Part model, mm, in its own coordinate system. A direction names the side the tool comes from. Round coordinates to 2 decimals unless told otherwise and drop trailing zeros. Loops run counter-clockwise (first coordinate to the right, second up) from the corner with the lowest first, then second, coordinate; pieces in that order, holes last.
(1) Probe probe 1 along Z at (x, y) = (148, 49.5) (3 decimals); probe 2 along Y at (x, z) = (171, -106); probe 3 along X at (y, z) = (-129, -416.5). List the from-to ranges inside material, lowest first.
(2) Cut at D-D on x = -84.5. List the corners of the cut face in (y, z) (3 decimals).
(3) Cut at C-C on z = -372.5. List the corners of the cut face in (x, y) (3 decimals), then the cut area to 3 significant figures.
(4) Cut at A-A on y = 0. List the corners of the cut face in (x, z) (3 decimals), then the cut area to 3 significant figures.
(5) Cut at B-B on z = -14.5. List the corners of the cut face in (x, y), then the cut area to 3 significant figures.
(6) Mould opens along X. For faces 1 (the face through (-228.6, -3, -308)), 2 (the face through (-118, 208.915, -504)), 3 (the face through (-86.949, -195.196, -145.643)), 4 (the face through (-84.531, -195.196, -471.703)) say: +X half, -X half, draft (parallel to the pull), parting line (faces both ways), or undercut.
(7) Tool access for faces 5 (the face through (238, -3, -624.205)), 6 (the face through (-128.216, 92.923, 123.657)), 7 (the face through (127, 431, -165.1)), 8 (the face through (-102, -200.025, -498)): list every direction of +Z, -Z, +X, -X, +Y, -Y with a clear straight run to the whole face (end or side of a thin tool).
(8) Flat gauge pins, fed straight in: pin 1 (1 mm diameter, centred on y = 207.5, z = -495, fed in from -X); pin 2 (21 mm diameter, centred on x = -20.5, y = -219, fed in from -Z) (3 decimals); pin 3 (6 mm diameter, centred on x = 39, z = -87.5, fed in from -Y). Where does each tip first touch, or does it go through?
from build123d import *

# Parameters (mm, degrees)
F0_W         = 457.2
F0_H         = 381
F1_DEPTH     = 625.475
F2_R         = 21.0935486288
F3_DEPTH     = 250.825
F4_R         = 21.4047690014
F5_DEPTH     = 209.55
F6_R         = 31.75
F6_R_2       = 1.5875
F6_R_3       = 6.35
F7_DEPTH     = 9.525
F8_W         = 19.05
F8_H         = 381
F9_DEPTH     = 76.2
F10_T1_DEPTH = 444.5
F12_R        = 96.52
F13_DEPTH    = 203.2
F15_DEPTH    = 12.7
F16_R        = 6.35
F17_DEPTH    = 266.7
F18_R        = 6.35
F19_DEPTH    = 114.3
F20_R        = 9.525
F21_DEPTH    = 170.18
F22_W        = 381
F22_H        = 1.27
F23_DEPTH    = 19.05
F24_W        = 381
F24_H        = 1.27
F25_DEPTH    = 19.05
F28_DEPTH    = 3.175


# Not quite as in the source:
# - a fillet or chamfer that OpenCascade refuses, or shapes differently, is made with other operations: its cross-section is extruded or revolved along the edge and cut away or added


with BuildPart() as f1:
    # F0 (on Top) → F1 (new body)
    with BuildSketch(Plane.XY):
        Rectangle(F0_W, F0_H)
    extrude(amount=-F1_DEPTH)

    # F2 (on face) → F3 (join)
    with BuildSketch(Plane.XY):
        with Locations((-125.4702359438, 72.0090046525)):
            Circle(F2_R)
    extrude(amount=F3_DEPTH)

    # F4 (on face) → F5 (join)
    with BuildSketch(Plane.XY):
        with Locations((-124.0155026317, 0)):
            Circle(F4_R)
    extrude(amount=F5_DEPTH)

    # F6 (on face) → F7 (join)
    with BuildSketch(Plane.XZ.offset(190.5)):
        with Locations((-101.6, -117.475)):
            Circle(F6_R)
        with Locations((-101.6, -498.475)):
            Circle(F6_R)
        with Locations((163.7871414423, -184.2048317194)):
            Circle(F6_R_2)
        with Locations((163.7871414423, -241.1169111729)):
            Circle(F6_R_3)
    extrude(amount=F7_DEPTH)

    # F8 (on face) → F9 (join)
    with BuildSketch(Plane.XZ.offset(190.5)):
        with Locations((-15.875, -307.975)):
            Rectangle(F8_W, F8_H)
    extrude(amount=F9_DEPTH)

    # F10: fillet of radius 12.7 on 2 edges, made by hand

    # F10_s2 → F10_t1 (cut)
    with BuildSketch(Plane.XY.offset(-530.225)):
        with BuildLine():
            ThreePointArc((-25.4, -254), (-21.6802561211, -262.9802561211), (-12.7, -266.7))
            Line((-12.7, -266.7), (-25.4, -266.7))
            Line((-25.4, -266.7), (-25.4, -254))
        make_face()
        with BuildLine():
            ThreePointArc((-6.35, -254), (-10.0697438789, -262.9802561211), (-19.05, -266.7))
            Line((-19.05, -266.7), (-6.35, -266.7))
            Line((-6.35, -266.7), (-6.35, -254))
        make_face()
    extrude(amount=F10_T1_DEPTH, mode=Mode.SUBTRACT)

    # F12 (on offset) → F13 (join)
    with BuildSketch(Plane.XY.offset(-152.4)):
        with Locations((127.0715296268, 284.48)):
            Circle(F12_R)
    extrude(amount=-F13_DEPTH)

    # F14 (on face) → F15 (join)
    with BuildSketch(Plane.XY.offset(-152.4)):
        Polygon((119.0875349175, 393.3692209579), (119.0875349175, 380.6692209579), (131.7875349175, 380.8847182149), (131.7875349175, 387.0192209579), (147.6625349175, 387.0192209579), (147.6625349175, 393.3692209579), (129.2475349175, 393.3692209579), (129.2475349175, 507.6692209579), (119.0875349175, 507.6692209579), align=None)
    extrude(amount=-F15_DEPTH)

    # F16 (on face) → F17 (join)
    with BuildSketch(Plane.XY.offset(-152.4)):
        with Locations((127.0715296268, 284.48)):
            Circle(F16_R)
    extrude(amount=F17_DEPTH)

    # F18 (on face) → F19 (join)
    with BuildSketch(Plane.XY):
        with Locations((127.4323694774, 125.7402606834)):
            Circle(F18_R)
    extrude(amount=F19_DEPTH)

    # F20 (on Right) → F21 (join, symmetric)
    with BuildSketch(Plane.YZ):
        with Locations((197.485, -555.625)):
            Circle(F20_R)
    extrude(amount=F21_DEPTH, both=True)

    # F22 (on face) → F23 (join)
    with BuildSketch(Plane(origin=(-228.6, 0, 0), x_dir=(0, -1, 0), z_dir=(-1, 0, 0))):
        with Locations((0, -624.84)):
            Rectangle(F22_W, F22_H)
    extrude(amount=F23_DEPTH)

    # F24 (on face) → F25 (join)
    with BuildSketch(Plane.YZ.offset(228.6)):
        with Locations((0, -624.84)):
            Rectangle(F24_W, F24_H)
    extrude(amount=F25_DEPTH)

    # F27 (on offset) → F28 (join)
    with BuildSketch(Plane.XZ.offset(-205.74)):
        with BuildLine():
            Line((-127, -555.625), (-107.95, -555.625))
            Line((-107.95, -555.625), (-107.95, -460.375))
            ThreePointArc((-107.95, -460.375), (-109.8098719395, -455.8848719395), (-114.3, -454.025))
            Line((-114.3, -454.025), (-120.65, -454.025))
            ThreePointArc((-120.65, -454.025), (-125.1401280605, -455.8848719395), (-127, -460.375))
            Line((-127, -460.375), (-127, -555.625))
        make_face()
    extrude(amount=-F28_DEPTH)


solid = f1.part
Final values:
1. probe 1: z = -625.475 to 0
1. probe 2: y = -190.5 to 190.5
1. probe 3: x = -228.6 to 228.6
2. outline: (-200.025, -525.227) - (-190.5, -525.227) - (-190.5, -625.475) - (190.5, -625.475) - (190.5, -562.101) arc R9.525 ccw (long way) to (190.5, -549.149) - (190.5, 0) - (-190.5, 0) - (-190.5, -90.723) - (-200.025, -90.723) - (-200.025, -144.227) - (-190.5, -144.227) - (-190.5, -471.723) - (-200.025, -471.723) - close
3. outline: (-228.6, -190.5) - (-25.4, -190.5) - (-25.4, -254) arc R12.7 ccw to (-15.875, -266.297) arc R12.7 ccw to (-6.35, -254) - (-6.35, -190.5) - (228.6, -190.5) - (228.6, 190.5) - (-228.6, 190.5) - close
3. area: 176,000 mm2
4. outline: (-247.65, -625.475) - (247.65, -625.475) - (247.65, -624.205) - (228.6, -624.205) - (228.6, 0) - (-102.611, 0) - (-102.611, 209.55) - (-145.42, 209.55) - (-145.42, 0) - (-228.6, 0) - (-228.6, -624.205) - (-247.65, -624.205) - close
4. area: 295,000 mm2
5. outline: (-228.6, -190.5) - (228.6, -190.5) - (228.6, 190.5) - (-228.6, 190.5) - close; circle Ø12.7 at (127.07, 284.48)
5. area: 174,000 mm2
6. face 1: -X half
6. face 2: draft
6. face 3: undercut
6. face 4: undercut
7. face 5: +Z, +X, +Y, -Y
7. face 6: +Z
7. face 7: -Z, +X, -X, +Y
7. face 8: +Z, -Z, -X, -Y
8. pin 1: stops at x = -127
8. pin 2: stops at z = -498.475
8. pin 3: stops at y = -190.5
